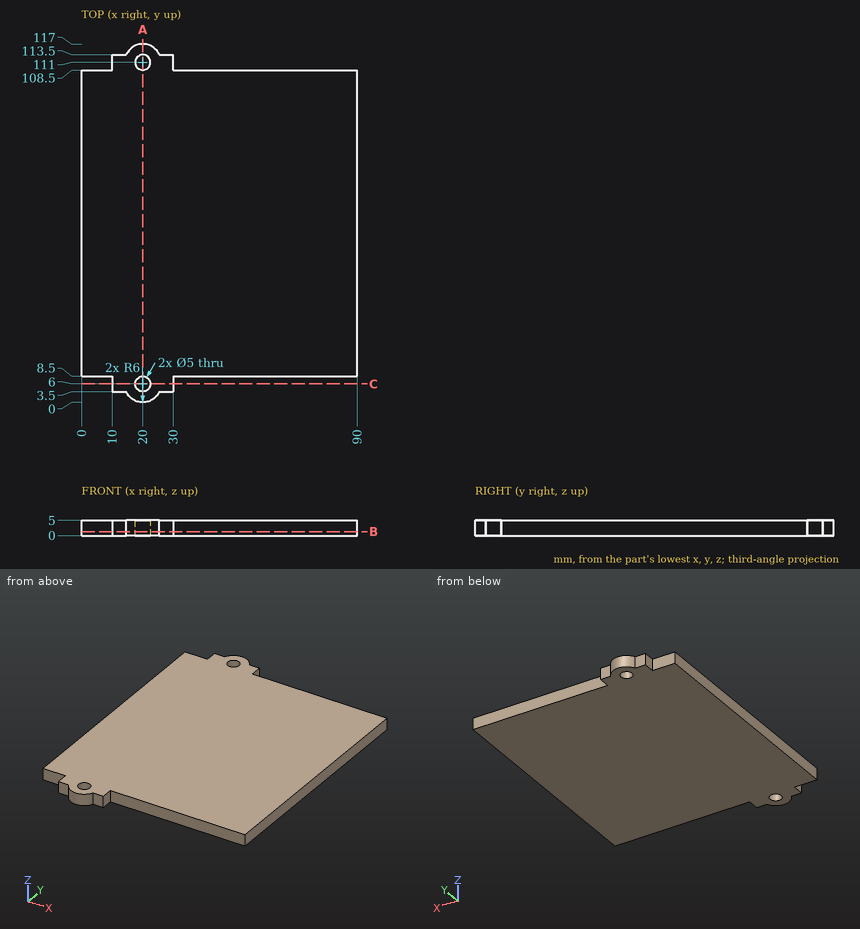
Verification items for this drawing (mm, ordinates from the low corner). Coordinates: 2 decimals unless noted, no trailing zeros. Loops run counter-clockwise (first coordinate to the right, second up) from the corner with the lowest first, then second, coordinate; pieces in that order, holes last. Notation, with made-up numbers: (-23.5, -11) -> (4.5, -11) arc R18 cw to (4.5, -2) -> close; hole circle Ø8 at (-17, 88). An arc over 180 degrees is marked (long way). Answer in a Markdown table with one row per item. Add a question column.
1. Material ranges on probe 1 along Y at (x, z) = (20, 3.45); probe 2 along Y at (x, z) = (22, 4.15); probe 3 along Y at (x, z) = (81.5, 2.1), recorded low to high. Write a range as [from, to].
2. Section check C-C, the plane y = 6. Enter the section's corners in (x, z), then the cut area to 3 significant figures.
3. Depth check by flat-ended pin: P1, Ø2.5, axis at x = 26.5, z = 2.5, coming from the -Y side; P2, Ø1.4, axis at x = 13, z = 2, coming from the +Y side; P3, Ø1.5, axis at y = 5, z = 3, coming from the +X side. Enter the tip coordinate at first touch or a pass-through.
4. Section check A-A, the plane x = 20. Enter the section's corners in (y, z).
5. Section check B-B, the plane z = 1.3. Enter the section's corners in (x, y).
Derived:
| question | item | result |
|---|---|---|
| 1 | probe 1 | y = [0, 3.5], [8.5, 108.5], [113.5, 117] |
| 1 | probe 2 | y = [0.34, 4.5], [7.5, 109.5], [112.5, 116.66] |
| 1 | probe 3 | y = [8.5, 108.5] |
| 2 | outline | (10, 0) -> (17.5, 0) -> (17.5, 5) -> (10, 5) -> close; (22.5, 0) -> (30, 0) -> (30, 5) -> (22.5, 5) -> close |
| 2 | area | 75.0 mm² |
| 3 | P1 | stops at y = 3.1 |
| 3 | P2 | stops at y = 113.5 |
| 3 | P3 | stops at x = 30 |
| 4 | outline | (0, 0) -> (3.5, 0) -> (3.5, 5) -> (0, 5) -> close; (8.5, 0) -> (108.5, 0) -> (108.5, 5) -> (8.5, 5) -> close; (113.5, 0) -> (117, 0) -> (117, 5) -> (113.5, 5) -> close |
| 5 | outline | (0, 8.5) -> (10, 8.5) -> (10, 3.5) -> (14.55, 3.5) arc R6 ccw to (25.45, 3.5) -> (30, 3.5) -> (30, 8.5) -> (90, 8.5) -> (90, 108.5) -> (30, 108.5) -> (30, 113.5) -> (25.45, 113.5) arc R6 ccw to (14.55, 113.5) -> (10, 113.5) -> (10, 108.5) -> (0, 108.5) -> close; hole circle Ø5 at (20, 6); hole circle Ø5 at (20, 111) |
